Can you work these out from the model? Positions are in its coordinate system, mm. Face numbers are marked on the shaded views. Round coordinates to 2 decimals unless told otherwise and drop trailing zeros. Write each loop counter-clockwise with the first axis right and the second up, starting at its lowest first coordinate (ties: lowest second). Pieces come first, ordered by that corner, then holes. Notation, with made-up numbers: M -6,-24 L 41,-24 A21 cw 41,10 Z; hole C 22.5,30 d1. An arc over 180 degrees is marked long. Answer as a JSON object with one key per item and string values. Group by question number.
1) I'm going to push a flat-ended pin straight in: pin 1 Ø8 at (x, y) = (-29.59, 4.94) entering from +Z. Where does the tip first touch, or does it pass through?
2) Suppose I cut it at A-A, the plane y = 0. Write out the boundary of the cut face in (x, z).
3) If we mould it in two halves opening along Z, with no side actions, what happens to the marked faces 1 and 2? For each: +Z half, -Z half, draft (parallel to the pull), parting line (faces both ways), or undercut.
4) Please list where these lines run through material, in increasing order: L1, parallel to Y at x = 29, z = 0.65; L2, parallel to X at y = -5, z = -0.7; L3, parallel to X at y = -11, z = 0.65. Write a range as [from, to].
5) Suppose I cut it at B-B, the plane z = 0.15. State how many separate pieces and enclosed holes the cut face has, and give its area (3 significant figures).
Autodesk Inventor part; units mm, degrees
ref_plane "YZ Plane" through (0, 0, 0) normal (1, 0, 0) x (0, 1, 0)
ref_plane "XZ Plane" through (0, 0, 0) normal (0, 1, 0) x (-1, 0, 0)
ref_plane "XY Plane" through (0, 0, 0) normal (0, 0, 1) x (1, 0, 0)
sketch "Sketch1" plane through (0, 0, 0) normal (0, 0, 1) x (1, 0, 0)
  circle A0 centre (0, 0) radius 25
  circle A1 centre (0, 0) radius 35
  circle A2 centre (30, 0) radius 3
  circle A3 centre (28.3745, 9.741) radius 3
  circle A4 centre (23.6742, 18.4264) radius 3
  circle A5 centre (16.4084, 25.115) radius 3
  circle A6 centre (7.3646, 29.082) radius 3
  circle A7 centre (-2.4774, 29.8975) radius 3
  circle A8 centre (-12.0509, 27.4732) radius 3
  circle A9 centre (-20.3184, 22.0717) radius 3
  circle A10 centre (-26.3842, 14.2784) radius 3
  circle A11 centre (-29.5908, 4.9378) radius 3
  circle A12 centre (-29.5908, -4.9378) radius 3
  circle A13 centre (-26.3842, -14.2784) radius 3
  circle A14 centre (-20.3184, -22.0717) radius 3
  circle A15 centre (-12.0509, -27.4732) radius 3
  circle A16 centre (-2.4774, -29.8975) radius 3
  circle A17 centre (7.3646, -29.082) radius 3
  circle A18 centre (16.4084, -25.115) radius 3
  circle A19 centre (23.6742, -18.4264) radius 3
  circle A20 centre (28.3745, -9.741) radius 3
  point P0 (35, 0)
  dimension "d2" = 70
  dimension "d0" = 50
  dimension "d3" = 6
  dimension "d4" = 5
  dimension "d7" = 360
extrude "Extrusion1" add sketch "Sketch1" along normal mid plane 1.6
chamfer "Chamfer1" distance 0.2 angle 45 42 edges at (20.6742, -18.4264, -0.8) (13.4084, -25.115, -0.8) (13.4084, -25.115, 0.8) (4.3646, -29.082, 0.8) (-15.0509, -27.4732, -0.8) (-15.0509, -27.4732, 0.8) (-5.4774, -29.8975, -0.8) (-5.4774, -29.8975, 0.8) (20.6742, -18.4264, 0.8) (4.3646, -29.082, -0.8) (25.3745, -9.741, -0.8) (25.3745, -9.741, 0.8) (-25, 0, -0.8) (-25, 0, 0.8) (-35, 0, -0.8) (-35, 0, 0.8) (-29.3842, 14.2784, -0.8) (-29.3842, 14.2784, 0.8) (-23.3184, 22.0717, -0.8) (-23.3184, 22.0717, 0.8) (20.6742, 18.4264, 0.8) (4.3646, 29.082, 0.8) (4.3646, 29.082, -0.8) (20.6742, 18.4264, -0.8) (-29.3842, -14.2784, -0.8) (-29.3842, -14.2784, 0.8) (-23.3184, -22.0717, -0.8) (-23.3184, -22.0717, 0.8) (-32.5908, -4.9378, 0.8) (-32.5908, -4.9378, -0.8) (-32.5908, 4.9378, -0.8) (-32.5908, 4.9378, 0.8) (27, 0, 0.8) (27, 0, -0.8) (-5.4774, 29.8975, -0.8) (-5.4774, 29.8975, 0.8) (13.4084, 25.115, -0.8) (13.4084, 25.115, 0.8) (25.3745, 9.741, -0.8) (25.3745, 9.741, 0.8) (-15.0509, 27.4732, -0.8) (-15.0509, 27.4732, 0.8)
properties part number "ballRing" material "Stainless Steel"
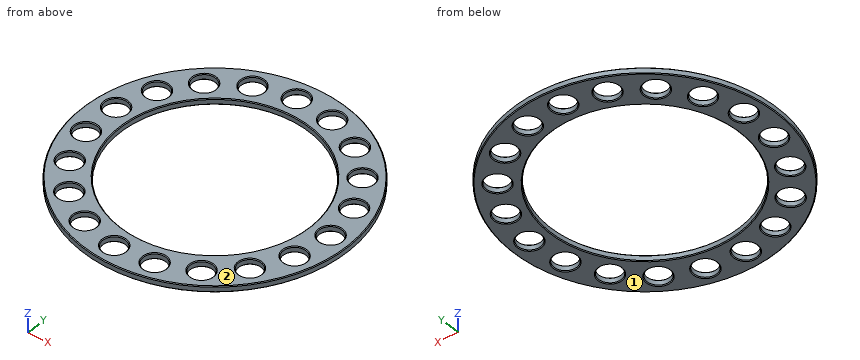
Results:
{
 "1": {"pin 1": "z = 0.8"},
 "2": {"outline": "M -35,-0.6 L -34.8,-0.8 L -25.2,-0.8 L -25,-0.6 L -25,0.6 L -25.2,0.8 L -34.8,0.8 L -35,0.6 Z; M 25,-0.6 L 25.2,-0.8 L 26.8,-0.8 L 27,-0.6 L 27,0.6 L 26.8,0.8 L 25.2,0.8 L 25,0.6 Z; M 33,-0.6 L 33.2,-0.8 L 34.8,-0.8 L 35,-0.6 L 35,0.6 L 34.8,0.8 L 33.2,0.8 L 33,0.6 Z"},
 "3": {"face 1": "-Z half", "face 2": "+Z half"},
 "4": {"L1": "[-19.51, -12.73], [-6.76, -2.88], [2.88, 6.76], [12.73, 19.51]", "L2": "[-34.54, -32.69], [-26.49, -24.6], [24.6, 34.54]", "L3": "[-33.17, -22.51], [22.51, 25.6], [31.15, 33.17]"},
 "5": {"separate pieces": "1", "enclosed holes": "20", "area": "1,350 mm^2"}
}
